Autodesk Fusion 360 part; units mm, degrees
sketch "Sketch1" plane through (0, 0, 0) normal (0, 0, 1) x (1, 0, 0)
  line L0 (0, 0) -> (-365.125, 0) construction
  line L1 (-365.125, 0) -> (-365.125, 47.244) construction
  line L2 (-365.125, 47.244) -> (0, 47.244) construction
  line L3 (0, 47.244) -> (0, -47.244) construction
  line L4 (0, -47.244) -> (-365.125, -47.244) construction
  line L5 (-365.125, -47.244) -> (-365.125, 47.244) construction
  line L6 (-47.244, 47.244) -> (-47.244, -47.244) construction
  arc A0 (-47.244, -47.244) -> (-47.244, 47.244) centre (-47.244, 0) ccw
  line L7 (-317.881, 47.244) -> (-317.881, -47.244) construction
  arc A1 (-317.881, 47.244) -> (-317.881, -47.244) centre (-317.881, 0) ccw
  line L8 (-317.881, 47.244) -> (-47.244, 47.244)
  line L9 (-47.244, -47.244) -> (-317.881, -47.244)
  line L10 (-365.125, -47.244) -> (-310.125, -47.244) construction
  line L11 (-310.125, -47.244) -> (-310.125, -17.244) construction
  line L12 (-310.125, -17.244) -> (-365.125, -17.244) construction
  line L13 (-365.125, -17.244) -> (-365.125, -47.244) construction
  circle A2 centre (-310.125, -17.244) radius 10
  dimension "d3" = 365.125
  dimension "d4" = 47.244
  dimension "d5" = 365.125
  dimension "d6" = 94.488
  dimension "d10" = 55
  dimension "d11" = 30
  dimension "d12" = 20
extrude "Extrude1" add sketch "Sketch1" along normal blind 2.9
sketch "Sketch2" plane through (0, 0, 0) normal (0, 0, -1) x (1, 0, 0)
  circle A0 centre (-310.125, 17.244) radius 10 construction
  arc A1 (-317.881, 47.244) -> (-317.881, -47.244) centre (-317.881, 0) ccw construction
  line L0 (-317.881, -47.244) -> (-47.244, -47.244) construction
  arc A2 (-47.244, -47.244) -> (-47.244, 47.244) centre (-47.244, 0) ccw construction
  line L1 (-47.244, 47.244) -> (-317.881, 47.244) construction
  line L2 (0, 0) -> (-365.125, 0) construction
  line L3 (0, 0) -> (-31, 0) construction
  line L4 (-31, 0) -> (-31, -100) construction
  line L5 (0, 0) -> (-52.5, 0) construction
  line L6 (-52.5, 0) -> (-52.5, -100) construction
  line L7 (-52.5, 0) -> (-44.5, 0) construction
  line L8 (-44.5, 0) -> (-44.5, -100) construction
  line L9 (-52.5, 0) -> (-40, 0) construction
  line L10 (-40, 0) -> (-40, -100) construction
  line L11 (-52.5, -47.244) -> (-52.5, -39.744) construction
  line L12 (-52.5, -39.744) -> (-52.5, -34.144) construction
  line L13 (-52.5, -39.744) -> (-52.5, -29.844) construction
  line L14 (-52.5, -39.744) -> (-52.5, -18.994) construction
  line L15 (-52.5, -39.744) -> (47.5, -39.744) construction
  line L16 (-52.5, -34.144) -> (47.5, -34.144) construction
  line L17 (-52.5, -29.844) -> (47.5, -29.844) construction
  line L18 (-52.5, -18.994) -> (47.5, -18.994) construction
  line L19 (-52.5, -39.744) -> (-317.881, -39.744)
  arc A3 (-52.5, -39.744) -> (-44.5, -34.144) centre (-53.3125, -30.069) ccw
  arc A4 (-40, -29.844) -> (-44.5, -34.144) centre (-36.8886, -37.6048) ccw
  arc A5 (-40, -29.844) -> (-31.5659, -21.0335) centre (-45.5992, -16.0418) ccw
  line L20 (0, 0) -> (-365.125, 0) construction
  arc A6 (-31.5659, 21.0335) -> (-40, 29.844) centre (-45.5992, 16.0418) ccw
  arc A7 (-44.5, 34.144) -> (-40, 29.844) centre (-36.8886, 37.6048) ccw
  arc A8 (-44.5, 34.144) -> (-52.5, 39.744) centre (-53.3125, 30.069) ccw
  line L21 (-52.5, 39.744) -> (-317.881, 39.744)
  line L22 (-31, -18.994) -> (-31, 18.994) construction
  line L23 (-317.881, -47.244) -> (-317.881, -39.744) construction
  line L24 (-365.125, 0) -> (-352.125, 0) construction
  arc A9 (-317.881, 39.744) -> (-317.881, -39.744) centre (-311.9393, 0) ccw
  line L25 (0, 0) -> (-13, 0) construction
  arc A10 (-28.8515, -18.7555) -> (-28.8515, 18.7555) centre (-32.0214, 0) ccw
  arc A11 (-28.8515, -18.7555) -> (-31.5659, -21.0335) centre (-28.2683, -22.2065) ccw
  arc A12 (-31.5659, 21.0335) -> (-28.8515, 18.7555) centre (-28.2683, 22.2065) ccw
  circle A13 centre (-310.125, 17.244) radius 10
  dimension "d22" = 31
  dimension "d23" = 52.5
  dimension "d24" = 100
  dimension "d25" = 100
  dimension "d26" = 8
  dimension "d27" = 100
  dimension "d28" = 12.5
  dimension "d29" = 100
  dimension "d34" = 7.5
  dimension "d35" = 5.6
  dimension "d36" = 9.9
  dimension "d37" = 20.75
  dimension "d38" = 100
  dimension "d39" = 100
  dimension "d40" = 100
  dimension "d41" = 100
  dimension "d42" = 7.5
  dimension "d43" = 13
  dimension "d44" = 13
  dimension "d45" = 3.5
extrude "Extrude2" add sketch "Sketch2" along normal blind 11
chamfer "Chamfer1" distance 0.7 angle 45 5 edges at (-182.5625, 47.244, 2.9) (-365.125, 0, 2.9) (-182.5625, -47.244, 2.9) (0, 0, 2.9) (-319.4483, -13.6278, 2.9)
chamfer "Chamfer1" distance 0.7 angle 45 13 edges at (-185.1905, -39.744, -11) (-352.125, 0, -11) (-47.7447, -38.023, -11) (-42.665, -31.5597, -11) (-34.8398, -26.3416, -11) (-34.8398, 26.3416, -11) (-30.5183, 19.5256, -11) (-13, 0, -11) (-30.5183, -19.5256, -11) (-42.665, 31.5597, -11) (-47.7447, 38.023, -11) (-185.1905, 39.744, -11) (-319.4483, -20.8602, -11)
sketch "Sketch3" plane through (0, -39.744, 0) normal (0, -1, 0) x (1, 0, 0)
  line L0 (-317.881, -10.3) -> (-52.5, -10.3)
  line L1 (-52.5, -10.3) -> (-52.5, 0)
  line L2 (-52.5, 0) -> (-317.881, 0)
  line L3 (-317.881, 0) -> (-317.881, -10.3)
  line L4 (-44.5, 0) -> (-40, 0)
  line L5 (-31.5659, 0) -> (-40, 0)
  line L6 (-31.5659, 0) -> (-28.8515, 0)
  line L7 (-13, 0) -> (-28.8515, 0)
  line L8 (-31.5659, 0) -> (-28.8515, 0)
  line L9 (-31.5659, 0) -> (-40, 0)
  line L10 (-44.5, 0) -> (-40, 0)
  line L11 (-44.5, 0) -> (-52.5, 0)
  line L12 (-52.5, 0) -> (-317.881, 0)
  line L13 (-317.881, 0) -> (-352.125, 0)
  line L14 (-317.881, 0) -> (-52.5, 0)
  line L15 (-44.5, 0) -> (-52.5, 0)
  line L16 (-317.881, 0) -> (-365.125, 0)
  line L17 (-317.881, 0) -> (-47.244, 0)
  line L18 (0, 0) -> (-47.244, 0)
  line L19 (-47.244, 0) -> (-317.881, 0)
  line L20 (-182.5625, 0) -> (-182.5625, -10.3) construction
  line L21 (-182.5625, 0) -> (-182.5625, -5.15) construction
hole "Hole1" at (-182.5625, -39.744, -5.15) direction (0, 1, 0) diameter 3.2 depth 20 tip angle 118 countersink diameter 8.5 countersink angle 90
ref_plane "WorkPlane1" through (-352.125, 0, 0) normal (1, 0, 0) x (0, 1, 0)
sketch "Sketch4" plane through (-352.125, 0, 0) normal (1, 0, 0) x (0, 1, 0)
  line L0 (39.044, -11) -> (-39.044, -11)
  line L1 (-39.744, 0) -> (39.744, 0)
  line L2 (0, 0) -> (0, -11)
  line L3 (0, 0) -> (0, -5.5)
hole "Hole2" at (-352.125, 0, -5.6194) direction (1, 0, 0) diameter 3.2 depth 20 tip angle 118 countersink diameter 8.5 countersink angle 90
equation "TopL = ( ( 14 + ( 3 / 8 ) ) * 25.4 ) * 1 mm"
equation "TopW = ( 3.72 * 25.4 ) * 1 mm"
equation "d3 = TopL"
equation "d4 = TopW / 2"
equation "d5 = TopL"
equation "d6 = TopW"
equation "HoleB = 30 mm"
equation "HoleR = 55 mm"
equation "HoleD = 20 mm"
equation "TopT = 2.9 mm"
equation "d14 = TopT"
equation "TrailEndO = 13 mm"
equation "TrailFC = 52.5 mm"
equation "TrailSC = 8 mm"
equation "TrailTC = 12.5 mm"
equation "TrailFlat = 31 mm"
equation "d22 = TrailFlat"
equation "d23 = TrailFC"
equation "d26 = TrailSC"
equation "d28 = TrailTC"
equation "TrailFW = 5.6 mm"
equation "TrailSW = 9.9 mm"
equation "TrailTW = 20.75 mm"
equation "BottomWO = 7.5 mm"
equation "d34 = BottomWO"
equation "d35 = TrailFW"
equation "d36 = TrailSW"
equation "d37 = TrailTW"
equation "d42 = BottomWO"
equation "d43 = TrailEndO"
equation "d44 = TrailEndO"
equation "BottomT = 11 mm"
equation "d47 = BottomT"
Input: part model. Units: mm. Frame: model coordinates. A direction names the side the tool comes from. Give positions to 0.01 mm unless a question says otherwise; leave off trailing zeros. Order: outer loops, then holes, each group sorted by start corner. A loop starts at its lowest first (then second) coordinate and runs counter-clockwise, first axis right, second up.
1. Section A-A on x = -153. Return the cut outline in (y, z).
Derived:
outline: (-47.24, 0) - (-39.74, 0) - (-39.74, -10.3) - (-39.04, -11) - (39.04, -11) - (39.74, -10.3) - (39.74, 0) - (47.24, 0) - (47.24, 2.2) - (46.54, 2.9) - (-46.54, 2.9) - (-47.24, 2.2) - close
2. Material intervals for L1, parallel to Z at x = -342.75, y = 0; L2, parallel to X at y = -12.5, z = -7.25; L3, parallel to X at y = -10.5, z = -0.5, sorted ascending.
Derived:
L1: z = -11 to -7.22, -4.02 to 2.9
L2: x = -350.13 to -318.93, -301.32 to -17.68
L3: x = -350.73 to -317.51, -302.74 to -16.16
3. Pin query (flat end, axial travel): pin 1 (18 mm diameter, centred on x = -310.125, y = -17.244, fed in from +Z); pin 2 (2 mm diameter, centred on y = 6, z = -4.5, fed in from +X); pin 3 (2.5 mm diameter, centred on x = -182.56, z = -5.15, fed in from -Y); pin 4 (5 mm diameter, centred on x = -155.5, z = -4, fed in from +Y). Return the tip coordinate at first contact, or that it passes through.
Derived:
pin 1: passes through
pin 2: stops at x = -13.67
pin 3: stops at y = -19.54
pin 4: stops at y = 39.74
4. Mould query, pull axis X, two halves, no side actions, for faces 6 (the cylindrical face through (-34.8, 26.3, -5.1)), 7 (the conical face through (-181.074, -37.26, -6.099)), 8 (the flat face through (-183, 39.744, -5)). Classes: released by +X, released by -X, zero draft, split by the parting line, or undercut.
Derived:
face 6: released by +X
face 7: undercut
face 8: zero draft
5. Reachability of faces 1 (the cylindrical face through (-34.901, -26.405, -5.078)), 2 (the cylindrical face through (-13, 0, -5)), 3 (the cylindrical face through (-352.117, 0.8, -0.5)), 4 (the flat face through (-170, -42, 0)), 5 (the flat face through (-183.3, -39.744, -0.5)) from +Z, -Z, +X, -X, +Y, -Y: full face, straight path, thin tool, end or side. Return the list, or none.
Derived:
face 1: -Z, +X, -Y
face 2: -Z, +X
face 3: -Z, -X
face 4: -Z
face 5: -Z, +X, -X, -Y
